Autodesk Inventor part; units mm, degrees
ref_plane "YZ Plane" through (0, 0, 0) normal (1, 0, 0) x (0, 1, 0)
ref_plane "XZ Plane" through (0, 0, 0) normal (0, 1, 0) x (-1, 0, 0)
ref_plane "XY Plane" through (0, 0, 0) normal (0, 0, 1) x (1, 0, 0)
sketch "Sketch1" plane through (0, 0, 0) normal (0, 0, 1) x (1, 0, 0)
  line L0 (0, 0) -> (25, 0)
  line L1 (25, 0) -> (25, 25)
  line L2 (25, 25) -> (0, 25)
  line L3 (0, 25) -> (0, 0)
  line L4 (3, 3) -> (22, 3)
  line L5 (22, 3) -> (22, 22)
  line L6 (22, 22) -> (3, 22)
  line L7 (3, 22) -> (3, 3)
  dimension "d0" = 25
  dimension "d1" = 25
  dimension "d2" = 3
extrude "Extrusion1" add sketch "Sketch1" along normal blind 500
sketch "Sketch3" plane through (25, 0, 0) normal (1, 0, 0) x (0, 0, -1)
  line L0 (0, 0) -> (0, 25)
  line L1 (0, 25) -> (-500, 25)
  line L2 (-500, 0) -> (-500, 25)
  line L3 (0, 0) -> (-500, 0)
  point P0 (0, 0)
  point P1 (-450, 12.5)
  point P2 (-50, 12.5)
  point P3 (-410, 12.5)
  point P4 (-370, 12.5)
  point P5 (-330, 12.5)
  point P6 (-290, 12.5)
  point P7 (-250, 12.5)
  point P8 (-210, 12.5)
  point P9 (-170, 12.5)
  point P10 (-130, 12.5)
  point P11 (-90, 12.5)
  dimension "d16" = 12.5
  dimension "d17" = 50
  dimension "d18" = 50
  dimension "d19" = 12.5
  dimension "d22" = 40
hole "Hole2" at (25, 12.5, 450) at (25, 12.5, 50) at (25, 12.5, 410) at (25, 12.5, 370) at (25, 12.5, 330) at (25, 12.5, 290) at (25, 12.5, 250) at (25, 12.5, 210) at (25, 12.5, 170) at (25, 12.5, 130) at (25, 12.5, 90) direction (-1, 0, 0) diameter 12 depth 8 tip angle 118
sketch "Sketch4" plane through (3, 3, 0) normal (1, 0, 0) x (0, 0, -1)
  circle A0 centre (-130, 9.5) radius 6
  circle A1 centre (-210, 9.5) radius 6
  circle A2 centre (-290, 9.5) radius 6
  circle A3 centre (-370, 9.5) radius 6
  circle A4 centre (-50, 9.5) radius 6
  circle A5 centre (-450, 9.5) radius 6
  circle A6 centre (-410, 9.5) radius 6
  circle A7 centre (-330, 9.5) radius 6
  circle A8 centre (-250, 9.5) radius 6
  circle A9 centre (-170, 9.5) radius 6
  circle A10 centre (-90, 9.5) radius 6
  line L0 (0, -3) -> (0, 22)
  line L1 (0, 22) -> (-500, 22)
  line L2 (-500, -3) -> (-500, 22)
  line L3 (0, -3) -> (-500, -3)
  arc A11 (0, -3) -> (0, -3) centre (-50, 9.5) ccw
  circle A12 centre (-210, 9.5) radius 6
  circle A13 centre (-250, 9.5) radius 6
  circle A14 centre (-370, 9.5) radius 6
  circle A15 centre (-410, 9.5) radius 6
hole "Hole3" at (3, 12.5, 50) at (3, 12.5, 90) at (3, 12.5, 130) at (3, 12.5, 170) at (3, 12.5, 210) at (3, 12.5, 250) at (3, 12.5, 290) at (3, 12.5, 330) at (3, 12.5, 370) at (3, 12.5, 410) at (3, 12.5, 450) direction (-1, 0, 0) diameter 7 depth 8 tip angle 118
sketch "Sketch6" plane through (0, 0, 0) normal (0, 0, -1) x (-1, 0, 0)
  line L0 (-25, 0) -> (-25, 25)
  line L1 (0, 0) -> (-25, 0)
  line L2 (0, 25) -> (0, 0)
  line L3 (-25, 25) -> (0, 25)
  line L4 (-3, 3) -> (-3, 22)
  line L5 (-22, 3) -> (-3, 3)
  line L6 (-22, 22) -> (-22, 3)
  line L7 (-3, 22) -> (-22, 22)
extrude "Extrusion3" add sketch "Sketch6" along normal blind 90
sketch "Sketch7" plane through (0, 0, 500) normal (-1, 0, 0) x (0, 0, 1)
  circle A0 centre (-90, 12.5) radius 3.5
  circle A1 centre (-170, 12.5) radius 3.5
  circle A2 centre (-250, 12.5) radius 3.5
  circle A3 centre (-330, 12.5) radius 3.5
  circle A4 centre (-410, 12.5) radius 3.5
  circle A5 centre (-450, 12.5) radius 3.5
  circle A6 centre (-370, 12.5) radius 3.5
  circle A7 centre (-290, 12.5) radius 3.5
  circle A8 centre (-210, 12.5) radius 3.5
  circle A9 centre (-130, 12.5) radius 3.5
  circle A10 centre (-50, 12.5) radius 3.5
  line L0 (-590, 0) -> (0, 0)
  line L1 (0, 25) -> (0, 0)
  line L2 (-590, 25) -> (0, 25)
  line L3 (-590, 0) -> (-590, 25)
  point P0 (-500, 0)
  point P1 (-577.5, 12.5)
  dimension "d47" = 12.5
  dimension "d48" = 12.5
hole "Hole4" at (0, 12.5, -77.5) direction (1, 0, 0) diameter 12 end through all
sketch "Sketch8" plane through (25, 0, 500) normal (1, 0, 0) x (0, 0, -1)
  point P0 (500, 0)
sketch "Sketch9" plane through (0, 0, 500) normal (-1, 0, 0) x (0, 0, 1)
  circle A0 centre (-577.5, 12.5) radius 6
  circle A1 centre (-90, 12.5) radius 3.5
  circle A2 centre (-170, 12.5) radius 3.5
  circle A3 centre (-250, 12.5) radius 3.5
  circle A4 centre (-330, 12.5) radius 3.5
  circle A5 centre (-410, 12.5) radius 3.5
  circle A6 centre (-450, 12.5) radius 3.5
  circle A7 centre (-370, 12.5) radius 3.5
  circle A8 centre (-290, 12.5) radius 3.5
  circle A9 centre (-210, 12.5) radius 3.5
  circle A10 centre (-130, 12.5) radius 3.5
  circle A11 centre (-50, 12.5) radius 3.5
  line L0 (-590, 0) -> (0, 0)
  line L1 (0, 25) -> (0, 0)
  line L2 (-590, 25) -> (0, 25)
  line L3 (-590, 0) -> (-590, 25)
  line L4 (0, 0) -> (0, 25)
  line L5 (0, 0) -> (-25, 25)
  line L6 (-590, 25) -> (0, 25)
  point P0 (-500, 0)
  dimension "d56" = 45
extrude "Extrusion4" cut sketch "Sketch9" against normal blind 109.75 contours L5 L2 L1
properties part number "P701" material "Aluminum 6061"
Source: CAD feature listing. Evaluate the final solid. Frame: model axes, mm. A direction names the side the tool comes from. Coordinates: 2 decimals unless noted, no trailing zeros. Write each loop counter-clockwise with the first axis right and the second up, starting at its lowest first coordinate (ties: lowest second). Pieces come first, ordered by that corner, then holes. Notation, with made-up numbers: (71.25, 24.5) -> (103.25, 24.5) arc R26 cw to (103.25, 41.5) -> close; hole circle Ø2 at (10, 17). An arc over 180 degrees is marked (long way). Return JSON: item names as keys, results as strings. Group by question number.
1) Mould query, pull axis X, two halves, no side actions, for faces 1 (the face through (13, 3, 208)), 2 (the face through (23, 12, 488)). Classes: +X half, -X half, draft (parallel to the pull), parting line (faces both ways), or undercut.
2) Set-up query: faces 3 (the face through (1.521, 12.236, -83.494)), 4 (the face through (12, 22, 198)), 5 (the face through (23.479, 12.236, 175.994)). Return all of +Z, -Z, +X, -X, +Y, -Y with unobstructed straight access to the full face (end or side cutting, diameter ignored); none if empty.
3) Ray query, line 1 along X through (y, z) = (20.75, 164.5); line 2 along Y through (x, z) = (1.8, 290). Return the intervals inside material, ascending.
4) Section query A-A, the plane x = 16.5. Return loops of the section in (y, z).
5) Contact query for flat-ended pins moving along their axis: P1, Ø6.5, axis at y = 12.5, z = 210, coming from the -X side; P2, Ø12, axis at x = 7.5, y = 16.5, coming from the +Z side. Output: stop coordinate, or through.
6) Section query B-B, the plane z = -11. Return loops of the section in (x, y).
From the geometry:
{
 "1": {"face 1": "undercut", "face 2": "draft"},
 "2": {"face 3": "+X, -X", "face 4": "+Z, -Z", "face 5": "+X"},
 "3": {"line 1": "0 to 3, 22 to 25", "line 2": "0 to 9, 16 to 25"},
 "4": {"outline": "(0, -90) -> (3, -90) -> (3, 497) -> (0, 500) -> close; (22, -90) -> (25, -90) -> (25, 475) -> (22, 478) -> close"},
 "5": {"P1": "through", "P2": "z = 487.47"},
 "6": {"outline": "(0, 0) -> (25, 0) -> (25, 25) -> (0, 25) -> close; hole (3, 3) -> (22, 3) -> (22, 22) -> (3, 22) -> close"}
}
